```python
from build123d import *

# Parameters (mm, degrees)
SKETCH5_W           = 146
SKETCH5_H           = 146
BOSS_EXTRUDE2_DEPTH = 250
FILLET8_R           = 40
FILLET9_R           = 40
FILLET10_R          = 40
FILLET11_R          = 40
FILLET12_R          = 10
BOSS_EXTRUDE5_START = -240
BOSS_EXTRUDE5_DEPTH = 240
SKETCH8_R           = 60
CUT_EXTRUDE1_DEPTH  = 34
SKETCH10_W          = 44
SKETCH10_H          = 33
CUT_EXTRUDE2_DEPTH  = 3
CUT_EXTRUDE3_DEPTH  = 3


# Read off the part's stored shape, not the designer's step: Boss-Extrude5
with BuildPart() as part:
    # Sketch5 → Boss-Extrude2 (new body)
    with BuildSketch(Plane(origin=(0, 0, 0), x_dir=(1, 0, 0), z_dir=(0, 1, 0))):
        Rectangle(SKETCH5_W, SKETCH5_H)
    extrude(amount=BOSS_EXTRUDE2_DEPTH)

    # Fillet8
    fillet8_edges = [part.edges().sort_by_distance(p)[0] for p in [
        (73, 125, 73),
    ]]
    fillet(fillet8_edges, radius=FILLET8_R)

    # Fillet9
    fillet9_edges = [part.edges().sort_by_distance(p)[0] for p in [
        (73, 125, -73),
    ]]
    fillet(fillet9_edges, radius=FILLET9_R)

    # Fillet10
    fillet10_edges = [part.edges().sort_by_distance(p)[0] for p in [
        (-73, 125, -73),
    ]]
    fillet(fillet10_edges, radius=FILLET10_R)

    # Fillet11
    fillet11_edges = [part.edges().sort_by_distance(p)[0] for p in [
        (-73, 125, 73),
    ]]
    fillet(fillet11_edges, radius=FILLET11_R)

    # Fillet12
    fillet12_edges = [part.edges().sort_by_distance(p)[0] for p in [
        (73, 250, 0),
        (61.284271247, 250, 61.284271247),
        (0, 250, -73),
        (61.284271247, 250, -61.284271247),
        (-73, 250, 0),
        (-61.284271247, 250, -61.284271247),
        (0, 250, 73),
        (-61.284271247, 250, 61.284271247),
    ]]
    fillet(fillet12_edges, radius=FILLET12_R)

    # Boss-Extrude5 outline → Boss-Extrude5 (cut)
    with BuildSketch(Plane.XZ.offset(BOSS_EXTRUDE5_START)):
        with BuildLine():
            Line((30, 70), (-30, 70))
            ThreePointArc((-30, 70), (-58.284271247, 58.284271247), (-70, 30))
            Line((-70, 30), (-70, -30))
            ThreePointArc((-70, -30), (-58.284271247, -58.284271247), (-30, -70))
            Line((-30, -70), (30, -70))
            ThreePointArc((30, -70), (58.284271247, -58.284271247), (70, -30))
            Line((70, -30), (70, 30))
            ThreePointArc((70, 30), (58.284271247, 58.284271247), (30, 70))
        make_face()
    extrude(amount=BOSS_EXTRUDE5_DEPTH, mode=Mode.SUBTRACT)

    # Sketch8 → Cut-Extrude1 (cut)
    with BuildSketch(Plane(origin=(0, 250, 0), x_dir=(1, 0, 0), z_dir=(0, 1, 0))):
        with Locations(Location((0, 0, 0), (0, 0, 270))):
            Circle(SKETCH8_R)
    extrude(amount=-CUT_EXTRUDE1_DEPTH, mode=Mode.SUBTRACT)

    # Sketch10 → Cut-Extrude2 (cut)
    with BuildSketch(Plane(origin=(73, 0, 0), x_dir=(0, 0, -1), z_dir=(1, 0, 0))):
        with Locations((0, 63.5)):
            Rectangle(SKETCH10_W, SKETCH10_H)
    extrude(amount=-CUT_EXTRUDE2_DEPTH, mode=Mode.SUBTRACT)

    # Sketch11 → Cut-Extrude3 (cut)
    with BuildSketch(Plane.ZY.offset(73)):
        Polygon((0, 0), (-16, 0), (-16, 13), (16, 13), (16, 0), align=None)
    extrude(amount=-CUT_EXTRUDE3_DEPTH, mode=Mode.SUBTRACT)


solid = part.part
```
Can you work these out from the model? Positions are in its coordinate system, mm. A direction names the side the tool comes from. Coordinates: 2 decimals unless noted, no trailing zeros. Loops run counter-clockwise (first coordinate to the right, second up) from the corner with the lowest first, then second, coordinate; pieces in that order, holes last. Notation, with made-up numbers: M -8.5,13 L 37.5,13 A11 ccw 37.5,25 Z; hole C -35,-30 d7. An arc over 180 degrees is marked long. Put each result on its own line as item: value. Start each with the question number.
(1) Imagine slicing it at D-D on x = 23.5. List the corners of the cut face in (y, z) for me, and give its area (3 significant figures).
(2) We'd pull the mould along X, two halves only. Please class faces 1 (the face through (70, 122, 0)), 2 (the face through (0, 118, 73)), 3 (the face through (-70.15, 246.99, 0.46)): +X half, -X half, draft (parallel to the pull), parting line (faces both ways), or undercut.
(3) Which directions (+Z, -Z, +X, -X, +Y, -Y) give clear straight access to the entire face, cutting with the end or side of a thin tool? Please do faces 4 (the face through (-70, 122, 0)), 5 (the face through (-11, 0, -71)).
(4) Imagine slicing it at A-A on z = 0. List the corners of the cut face in (x, y) for me, and give its area (3 significant figures).
(5) Will these pins go through, and if not, where does the flat tip stop? pin 1 Ø2.5 at (x, y) = (-71, 7) entering from -Z; pin 2 Ø2.5 at (x, z) = (71.5, 6) entering from +Y; pin 3 Ø5 at (y, z) = (128.5, 43) entering from -X.
(6) Imagine slicing it at B-B on y = 168.5. List the corners of the cut face in (x, z) for me, and give its area (3 significant figures).
(7) I need wall thicknesses on probe 1 along X at (y, z) = (218.5, 8.5); probe 2 along X at (y, z) = (127, 32). Which ranges of each line are inside material? Lowest first, please.
(8) Imagine slicing it at C-C on x = 0. List the corners of the cut face in (y, z) for me.
Worked answers:
1. outline: M 0,-73 L 240,-73 A10 ccw 250,-63 L 250,-55.21 L 240,-55.21 L 240,-70 L 0,-70 Z; M 0,70 L 240,70 L 240,55.21 L 250,55.21 L 250,63 A10 ccw 240,73 L 0,73 Z
1. area: 1,750 mm2
2. face 1: undercut
2. face 2: draft
2. face 3: -X half
3. face 4: -Y
3. face 5: +Z, -Z, +X, -X, -Y
4. outline: M -73,13 L -70,13 L -70,240 L -60,240 L -60,250 L -63,250 A10 ccw -73,240 Z; M 60,240 L 70,240 L 70,80 L 73,80 L 73,240 A10 ccw 63,250 L 60,250 Z; M 70,0 L 73,0 L 73,47 L 70,47 Z
4. area: 1,520 mm2
5. pin 1: stops at z = -48.79
5. pin 2: stops at y = 246.89
5. pin 3: stops at x = -72.29
6. outline: M -73,-33 A40 ccw -33,-73 L 33,-73 A40 ccw 73,-33 L 73,33 A40 ccw 33,73 L -33,73 A40 ccw -73,33 Z; hole M -70,-30 A40 ccw -30,-70 L 30,-70 A40 ccw 70,-30 L 70,30 A40 ccw 30,70 L -30,70 A40 ccw -70,30 Z
6. area: 1,720 mm2
7. probe 1: x = -73 to -70, 70 to 73
7. probe 2: x = -73 to -69.95, 69.95 to 73
8. outline: M 0,-73 L 240,-73 A10 ccw 250,-63 L 250,-60 L 240,-60 L 240,-70 L 0,-70 Z; M 0,70 L 240,70 L 240,60 L 250,60 L 250,63 A10 ccw 240,73 L 0,73 Z
